Check sheet for the drawn part. Datum: minimum x, y, z corner. Units: mm. Coordinates: 2 decimals unless noted, no trailing zeros. Write each loop counter-clockwise with the first axis right and the second up, starting at its lowest first coordinate (ties: lowest second). Pieces come first, ordered by that corner, then holes. Notation, with made-up numbers: M -31.75,68 L 26.25,68 A32 ccw 26.25,101 Z; hole C 12.5,71.5 d8. An arc over 180 degrees is marked long. Answer in a Markdown table with one row per item.
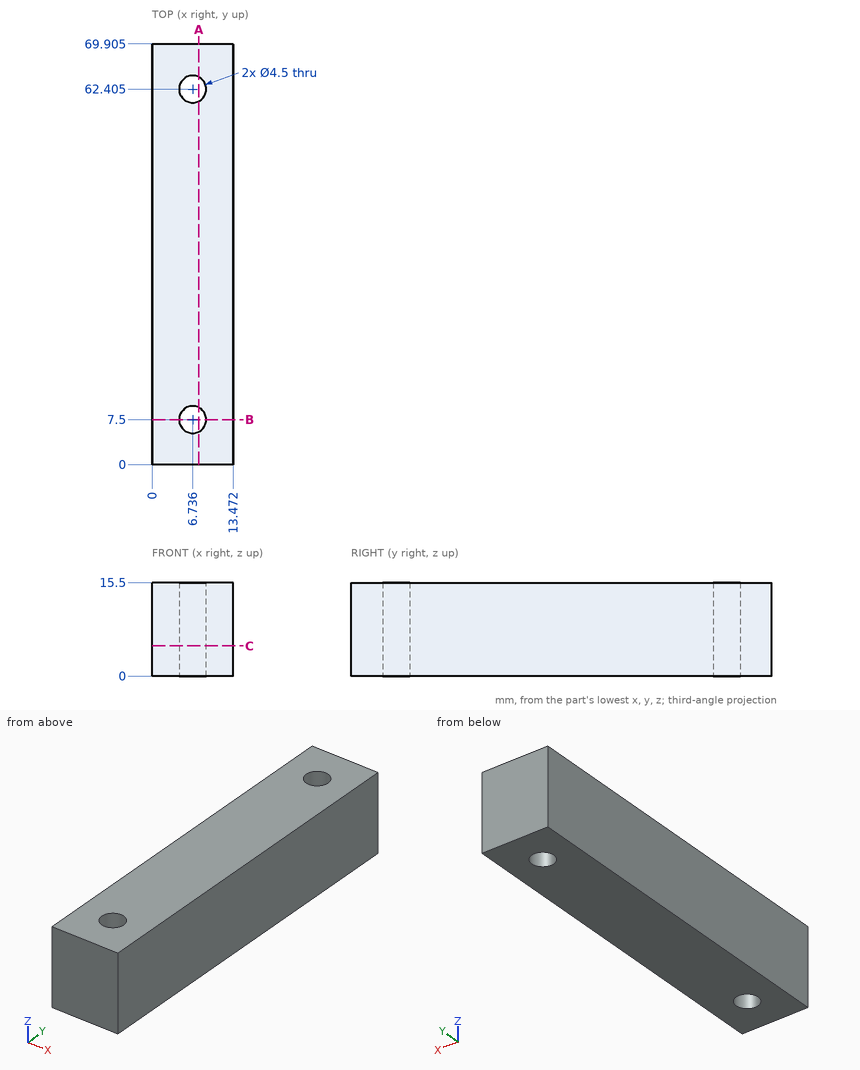
1) Sectioned sample at B-B (y = 7.5). Record the cut outline in (x, z).
Response values:
| item | result |
|---|---|
| outline | M 0,0 L 4.49,0 L 4.49,15.5 L 0,15.5 Z; M 8.99,0 L 13.47,0 L 13.47,15.5 L 8.99,15.5 Z |
2) Thickness scan on L1, parallel to Y at x = 6.5, z = 10.25 (1 decimal); L2, parallel to Y at x = 7.75, z = 6.5 (1 decimal). Record the ranges inside material, lowest first. Write a range as [from, to].
Response values:
| item | result |
|---|---|
| L1 | y = [0, 5.3], [9.7, 60.2], [64.6, 69.9] |
| L2 | y = [0, 5.5], [9.5, 60.4], [64.4, 69.9] |
3) Sectioned sample at C-C (z = 5). Give the number of separate pieces and of enclosed holes in the cut face, then the cut area to 3 significant figures.
Response values:
| item | result |
|---|---|
| separate pieces | 1 |
| enclosed holes | 2 |
| area | 910 mm² |
4) Sectioned sample at A-A (x = 7.75). Record the cut outline in (y, z) (1 decimal).
Response values:
| item | result |
|---|---|
| outline | M 0,0 L 5.5,0 L 5.5,15.5 L 0,15.5 Z; M 9.5,0 L 60.4,0 L 60.4,15.5 L 9.5,15.5 Z; M 64.4,0 L 69.9,0 L 69.9,15.5 L 64.4,15.5 Z |
